Verification items for the finished model (mm, model axes). Face numbers are marked on the shaded views. A direction names the side the tool comes from. Give positions to 0.01 mm unless a question says otherwise; leave off trailing zeros. Order: outer loops, then holes, each group sorted by start corner. A loop starts at its lowest first (then second) coordinate and runs counter-clockwise, first axis right, second up.
(1) Scan lines: L1, parallel to Z at x = 0, y = -13.75; L2, parallel to X at y = -16, z = 1; L3, parallel to X at y = -17.75, z = 49.5. Record each from-to range of solid material in increasing order.
(2) Gauge pin test, flat end, axial feed: pin 1 (7.5 mm diameter, centred on x = 27.5, y = -16, fed in from +Z). Record the tip position at first contact, or that the pin passes through.
(3) Access from +Z, -Z, +X, -X, +Y, -Y to the whole of each face (thin tool, end or side, straight path). Record for the marked faces 1 and 2.
(4) Sectioned sample at B-B on x = 0. Record the cut outline in (y, z), plus the area to 3 significant figures.
(5) Mould release check, pull along X, two halves, no side actions. Record for the marked faces 3, 4 and 5: pulls with the +X half, pulls with the -X half, needs draft (parallel to the pull), parting line crosses it, or undercut.
(6) Sectioned sample at D-D on y = -14.25. Record the cut outline in (x, z), plus the area to 3 significant figures.
(7) Sectioned sample at C-C on y = -1.75. Record the cut outline in (x, z), plus the area to 3 significant figures.
(8) Sectioned sample at A-A on z = 0. Record the cut outline in (x, y), plus the area to 3 significant figures.
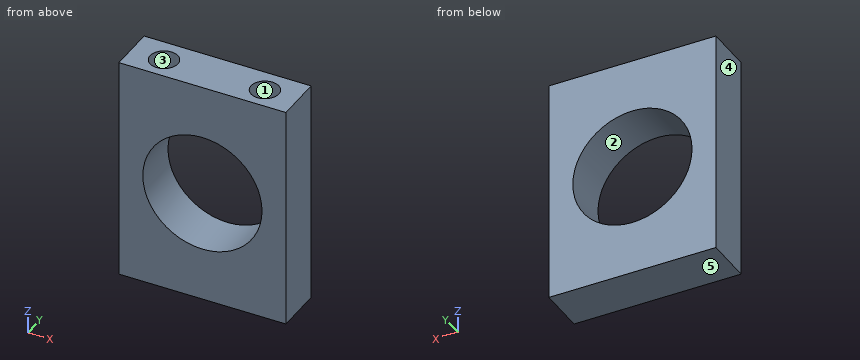
```python
from build123d import *

# Parameters (mm, degrees)
F0_W     = 88.246942
F0_H     = 119.301722
F1_DEPTH = 25
F3_R     = 7.34388
F4_DEPTH = 15
F2_R     = 31.491044
F5_DEPTH = 25


with BuildPart() as f1:
    # F0 (on Front) → F1 (new body)
    with BuildSketch(Plane.XZ):
        Rectangle(F0_W, F0_H)
    extrude(amount=F1_DEPTH)

    # F3 (on face) → F4 (cut)
    with BuildSketch(Plane.XY.offset(59.650861)):
        with Locations((-26.653793, -13.027571)):
            Circle(F3_R)
        with Locations((26.653793, -13.027571)):
            Circle(F3_R)
    extrude(amount=-F4_DEPTH, mode=Mode.SUBTRACT)

    # F2 (on face) → F5 (cut, through all)
    with BuildSketch(Plane.XZ.offset(25)):
        Circle(F2_R)
    extrude(amount=-F5_DEPTH, mode=Mode.SUBTRACT)


solid = f1.part
```
Ans:
1. L1: z = -59.65 to -31.49, 31.49 to 59.65
1. L2: x = -44.12 to -31.48, 31.48 to 44.12
1. L3: x = -44.12 to -32.28, -21.03 to 21.03, 32.28 to 44.12
2. pin 1: stops at z = 44.65
3. face 1: +Z
3. face 2: +Y, -Y
4. outline: (-25, -59.65) - (0, -59.65) - (0, -31.49) - (-25, -31.49) - close; (-25, 31.49) - (0, 31.49) - (0, 59.65) - (-25, 59.65) - close
4. area: 1,410 mm2
5. face 3: undercut
5. face 4: pulls with the -X half
5. face 5: needs draft
6. outline: (-44.12, -59.65) - (44.12, -59.65) - (44.12, 59.65) - (33.9, 59.65) - (33.9, 44.65) - (19.41, 44.65) - (19.41, 59.65) - (-19.41, 59.65) - (-19.41, 44.65) - (-33.9, 44.65) - (-33.9, 59.65) - (-44.12, 59.65) - close; hole circle Ø62.98 at (0, 0)
6. area: 6,980 mm2
7. outline: (-44.12, -59.65) - (44.12, -59.65) - (44.12, 59.65) - (-44.12, 59.65) - close; hole circle Ø62.98 at (0, 0)
7. area: 7,410 mm2
8. outline: (-44.12, -25) - (-31.49, -25) - (-31.49, 0) - (-44.12, 0) - close; (31.49, -25) - (44.12, -25) - (44.12, 0) - (31.49, 0) - close
8. area: 632 mm2
